The model under review builds one solid part; all positions refer to its coordinate system, in mm. Give positions to 0.01 mm unless a question says otherwise; leave off trailing zeros. Order: outer loops, then holes, each group sorted by start corner. A loop starts at its lowest first (then second) coordinate and runs counter-clockwise, first axis right, second up. Notation, with made-up numbers: (56.5, 6) -> (105.5, 6) arc R11 cw to (105.5, 22) -> close; hole circle Ø10 at (-28.5, -8.5). An arc over 180 degrees is marked (long way). Use one line per item in the form item = value.
```python
from build123d import *

# Parameters (mm, degrees)
F1_DEPTH = 9


with BuildPart() as f1:
    # F0 (on Top) → F1 (new body)
    with BuildSketch(Plane.XY):
        with BuildLine():
            Line((15, -51), (15, 0))
            ThreePointArc((15, 0), (0, 15), (-15, 0))
            Line((-15, 0), (-15, -51))
            Line((-15, -51), (-6, -60))
            Line((-6, -60), (6, -60))
            Line((6, -60), (15, -51))
        make_face()
    extrude(amount=F1_DEPTH)


solid = f1.part
```
1. For L1, parallel to Y at x = -0.5, z = 4.5; L2, parallel to Y at x = 2.5, z = 2.25; L3, parallel to X at y = -56, z = 6.5, list the stretches that pass through material, from the lowest coordinate up.
Values:
L1 = -60 to 14.99
L2 = -60 to 14.79
L3 = -10 to 10
2. For pin 1 Ø2 at (x, z) = (-10, 2.5) entering from +Y; pin 2 Ø4 at (x, z) = (4, 3) entering from +Y; pin 3 Ø1 at (x, z) = (10.5, 3.5) entering from +Y, all flat-tipped, find the tip position at first contact; note any pin that passes through.
Values:
pin_1 = 12
pin_2 = 14.87
pin_3 = 11.18
3. Add section B-B on x = 9. Give the boundary of the cut face in (y, z), then the cut area to 3 significant figures.
Values:
outline = (-57, 0) -> (12, 0) -> (12, 9) -> (-57, 9) -> close
area = 621 mm^2
4. Add section C-C on x = 12.25. Give the boundary of the cut face in (y, z).
Values:
outline = (-53.75, 0) -> (8.66, 0) -> (8.66, 9) -> (-53.75, 9) -> close
5. Add section A-A on z = 4. Give the boundary of the cut face in (x, y).
Values:
outline = (-15, -51) -> (-6, -60) -> (6, -60) -> (15, -51) -> (15, 0) arc R15 ccw to (-15, 0) -> close
